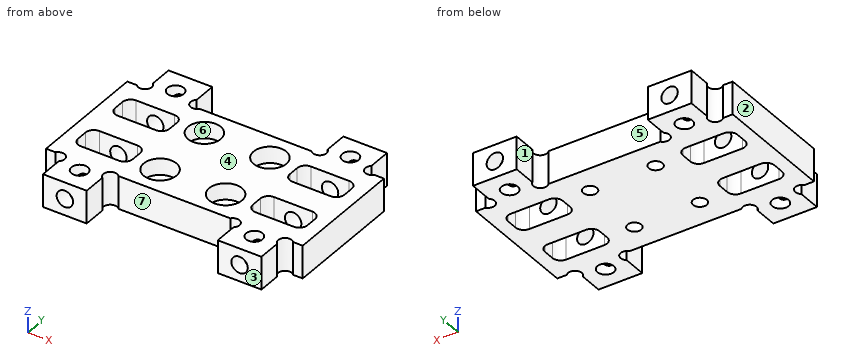
```python
from build123d import *

# Parameters (mm, degrees)
EXTRUDE_1_DEPTH          = 6
CUT_EXTRUDE_1_DEPTH      = 10
CUT_EXTRUDE_1_DEPTH_BACK = 38.043892884
SKETCH_3_R               = 1.5
SKETCH_4_W               = 10
SKETCH_4_H               = 5
CUT_EXTRUDE_2_DEPTH      = 30.618406439
SKETCH_5_R               = 1.5
CUT_EXTRUDE_3_DEPTH      = 30.618406439
FILLET_4_R               = 1.5
SKETCH_9_R               = 1.25
CUT_EXTRUDE_7_DEPTH      = 30.618406439
SKETCH_11_R              = 1.25
CUT_EXTRUDE_9_DEPTH      = 30.618406439
SKETCH_12_R              = 3
CUT_EXTRUDE_10_DEPTH     = 3


with BuildPart() as part:
    # 草图1 → 凸台-拉伸1 (new body)
    with BuildSketch(Plane.XY):
        Polygon((-23.5, 11), (-20, 11), (-20, 17), (-12, 17), (-12, 11), (12, 11), (12, 17), (20, 17), (20, 11), (23.5, 11), (23.5, -11), (20, -11), (20, -17), (12, -17), (12, -11), (-12, -11), (-12, -17), (-20, -17), (-20, -11), (-23.5, -11), align=None)
    extrude(amount=EXTRUDE_1_DEPTH)

    # 草图3 → 切除-拉伸1 (cut, two sides: drawn at the far end of the back side and taken through both)
    with BuildSketch(Plane(origin=(0, 11, 0), x_dir=(1, 0, 0), z_dir=(0, 1, 0)).offset(-CUT_EXTRUDE_1_DEPTH_BACK)):
        with Locations(Location((16, -3, 0), (0, 0, 90))):
            Circle(SKETCH_3_R)
        with Locations(Location((-16, -3, 0), (0, 0, 90))):
            Circle(SKETCH_3_R)
    extrude(amount=CUT_EXTRUDE_1_DEPTH + CUT_EXTRUDE_1_DEPTH_BACK, mode=Mode.SUBTRACT)

    # 草图4 → 切除-拉伸2 (cut, through all)
    with BuildSketch(Plane(origin=(0, 0, 0), x_dir=(-1, 0, 0), z_dir=(0, 0, -1))):
        with Locations((16, 5)):
            Rectangle(SKETCH_4_W, SKETCH_4_H)
        with Locations((16, -5)):
            Rectangle(SKETCH_4_W, SKETCH_4_H)
        with Locations((-16, 5)):
            Rectangle(SKETCH_4_W, SKETCH_4_H)
        with Locations((-16, -5)):
            Rectangle(SKETCH_4_W, SKETCH_4_H)
    extrude(amount=-CUT_EXTRUDE_2_DEPTH, mode=Mode.SUBTRACT)

    # 草图5 → 切除-拉伸3 (cut, through all)
    with BuildSketch(Plane(origin=(0, 0, 0), x_dir=(-1, 0, 0), z_dir=(0, 0, -1))):
        with Locations((-16, 13)):
            Circle(SKETCH_5_R)
        with Locations(Location((16, 13, 0), (0, 0, 180))):
            Circle(SKETCH_5_R)
        with Locations((16, -13)):
            Circle(SKETCH_5_R)
        with Locations(Location((-16, -13, 0), (0, 0, 180))):
            Circle(SKETCH_5_R)
    extrude(amount=-CUT_EXTRUDE_3_DEPTH, mode=Mode.SUBTRACT)

    # 圆角4
    fillet_4_edges = [part.edges().sort_by_distance(p)[0] for p in [
        (21, -7.5, 3),
        (21, -2.5, 3),
        (11, -2.5, 3),
        (11, -7.5, 3),
        (21, 2.5, 3),
        (21, 7.5, 3),
        (11, 7.5, 3),
        (11, 2.5, 3),
        (-11, -7.5, 3),
        (-11, -2.5, 3),
        (-21, -2.5, 3),
        (-21, -7.5, 3),
        (-11, 7.5, 3),
        (-21, 7.5, 3),
        (-21, 2.5, 3),
        (-11, 2.5, 3),
    ]]
    fillet(fillet_4_edges, radius=FILLET_4_R)

    # 草图9 → 切除-拉伸7 (cut, through all)
    with BuildSketch(Plane(origin=(0, 0, 0), x_dir=(-1, 0, 0), z_dir=(0, 0, -1))):
        with Locations((-11.2, 11.8)):
            Circle(SKETCH_9_R)
        with Locations((11.2, 11.8)):
            Circle(SKETCH_9_R)
        with Locations((11.2, -11.8)):
            Circle(SKETCH_9_R)
        with Locations((-11.2, -11.8)):
            Circle(SKETCH_9_R)
        with Locations((-20.8, 11.8)):
            Circle(SKETCH_9_R)
        with Locations((20.8, 11.8)):
            Circle(SKETCH_9_R)
        with Locations((20.8, -11.8)):
            Circle(SKETCH_9_R)
        with Locations((-20.8, -11.8)):
            Circle(SKETCH_9_R)
    extrude(amount=-CUT_EXTRUDE_7_DEPTH, mode=Mode.SUBTRACT)

    # 草图11 → 切除-拉伸9 (cut, through all)
    with BuildSketch(Plane(origin=(0, 0, 0), x_dir=(-1, 0, 0), z_dir=(0, 0, -1))):
        with Locations((6, 6)):
            Circle(SKETCH_11_R)
        with Locations((6, -6)):
            Circle(SKETCH_11_R)
        with Locations(Location((-6, 6, 0), (0, 0, 180))):
            Circle(SKETCH_11_R)
        with Locations(Location((-6, -6, 0), (0, 0, 180))):
            Circle(SKETCH_11_R)
    extrude(amount=-CUT_EXTRUDE_9_DEPTH, mode=Mode.SUBTRACT)

    # 草图12 → 切除-拉伸10 (cut)
    with BuildSketch(Plane.XY.offset(6)):
        with Locations((-6, 6)):
            Circle(SKETCH_12_R)
        with Locations((-6, -6)):
            Circle(SKETCH_12_R)
        with Locations((6, 6)):
            Circle(SKETCH_12_R)
        with Locations((6, -6)):
            Circle(SKETCH_12_R)
    extrude(amount=-CUT_EXTRUDE_10_DEPTH, mode=Mode.SUBTRACT)


solid = part.part
```
Build history of the part. All positions in model axes, mm. Face numbers are marked on the shaded views. A direction names the side the tool comes from. Round coordinates to 2 decimals unless told otherwise and drop trailing zeros. Write each loop counter-clockwise with the first axis right and the second up, starting at its lowest first coordinate (ties: lowest second). Pieces come first, ordered by that corner, then holes.
1) Band-saw the part on C-C, the plane y = 1.5. List the corners of the cut face in (x, z).
2) Band-saw the part on A-A, the plane x = 19. List the corners of the cut face in (y, z).
3) Mould opens along X. For the marked faces 1, 2 and 3 say: +X half, -X half, draft (parallel to the pull), parting line (faces both ways), or undercut.
4) Drill centre lines: probe 1 along X at (y, z) = (13, 1.5); probe 2 along Y at (x, z) = (18, 5.15); probe 3 along Z at (x, y) = (16, 14.65). Where is each one in solid material? Low to high.
5) 3-axis set-ups, long thin cutter, end or side, ignore diameter. For the marked faces 4, 5, 6 and 7: which of +Z, -Z, +X, -X, +Y, -Y reach the whole face in a straight line?
6) Pin check, flat tips, straight feed: pin 1 (1.8 mm diameter, centred on x = -5, z = 3.5, fed in from +Y); pin 2 (2 mm diameter, centred on y = -15, z = 3.5, fed in from -X). Stop position of each tip, or through.
7) Band-saw the part on B-B, the plane z = 2.25. Give the number of separate pieces and of enclosed holes in the cut face, and give its area (3 significant figures).
Ans:
1. outline: (-23.5, 0) - (23.5, 0) - (23.5, 6) - (-23.5, 6) - close; hole circle Ø3 at (-16, 3); hole circle Ø3 at (16, 3)
2. outline: (-17, 0) - (-7.5, 0) - (-7.5, 6) - (-17, 6) - close; (-2.5, 0) - (2.5, 0) - (2.5, 6) - (-2.5, 6) - close; (7.5, 0) - (17, 0) - (17, 6) - (7.5, 6) - close
3. face 1: undercut
3. face 2: -X half
3. face 3: draft
4. probe 1: x = -20 to -17.5, -14.5 to -12, 12 to 14.5, 17.5 to 20
4. probe 2: y = -17 to -7.5, -2.5 to 2.5, 7.5 to 17
4. probe 3: z = 0 to 1.5, 4.5 to 6
5. face 4: +Z, +X, -X, +Y, -Y
5. face 5: +Z, -Z, +Y
5. face 6: +Z
5. face 7: +Z, -Z, -Y
6. pin 1: stops at y = 11
6. pin 2: stops at x = -20
7. separate pieces: 3
7. enclosed holes: 4
7. area: 878 mm2
